```python
from build123d import *

# Parameters (mm, degrees)
BOSS_EXTRUDE1_DEPTH              = 6
FILLET1_R                        = 20
FILLET2_R                        = 20
SKETCH30_R                       = 10
CUT_EXTRUDE44_DEPTH              = 7
CUT_EXTRUDE44_DEPTH_BACK         = 1
SKETCH31_R                       = 5
CUT_EXTRUDE45_DEPTH              = 10
BODY_MOVE_COPY3_ANGLE            = 90
BODY_MOVE_COPY4_ANGLE            = 180
F_10_0MM_DOWEL_HOLE1_D           = 10
F_10_0MM_DOWEL_HOLE1_DEPTH       = 50
F_10_0MM_DOWEL_HOLE1_CSINK_D     = 10.05
F_10_0MM_DOWEL_HOLE1_CSINK_ANGLE = 90
F_10_0MM_DOWEL_HOLE1_TIP         = 3.004303095
SKETCH35_W                       = 43.4
SKETCH35_H                       = 43.4
CUT_EXTRUDE46_DEPTH              = 200


with BuildPart() as part:
    # Sketch6 → Boss-Extrude1 (new body)
    with BuildSketch(Plane.XY):
        Polygon((-61.363636364, 0), (61.363636364, 0), (90.231149823, -50), (90.231149823, -115), (54.237430104, -170), (54.237430104, -290), (-56.622130409, -290), (-56.622130409, -170), (-89.768850177, -115), (-89.768850177, -50), align=None)
    extrude(amount=BOSS_EXTRUDE1_DEPTH)

    # Fillet1
    fillet1_edges = [part.edges().sort_by_distance(p)[0] for p in [
        (54.237430104, -290, 3),
    ]]
    fillet(fillet1_edges, radius=FILLET1_R)

    # Fillet2
    fillet2_edges = [part.edges().sort_by_distance(p)[0] for p in [
        (-56.622130409, -290, 3),
    ]]
    fillet(fillet2_edges, radius=FILLET2_R)

    # Sketch30 → Cut-Extrude44 (cut, two sides)
    with BuildSketch(Plane.XY) as cut_extrude44_sk:
        with Locations((-1.192350152, -220)):
            Circle(SKETCH30_R)
    extrude(amount=CUT_EXTRUDE44_DEPTH, mode=Mode.SUBTRACT)
    extrude(cut_extrude44_sk.sketch, amount=-CUT_EXTRUDE44_DEPTH_BACK, mode=Mode.SUBTRACT)

    # Sketch31 → Cut-Extrude45 (cut)
    with BuildSketch(Plane.XY.offset(6)):
        with Locations((0, -69.133646514)):
            Circle(SKETCH31_R)
    extrude(amount=-CUT_EXTRUDE45_DEPTH, mode=Mode.SUBTRACT)


with BuildPart() as part_1:
    # Body-Move/Copy3: moved
    add(part.part.rotate(Axis((0, -121.936798964, -1), (1, 0, 0)), BODY_MOVE_COPY3_ANGLE))


with BuildPart() as part_2:
    # Body-Move/Copy4: moved
    add(part_1.part.rotate(Axis((0, -111.936798964, -21), (1, 0, 0)), BODY_MOVE_COPY4_ANGLE))


with BuildPart() as part_3:
    # Body-Move/Copy5: moved
    add(part_2.part.moved(Location((52.144140366, 0, 0))))

    # Ø10.0mm Dowel Hole1
    with Locations(Plane(origin=(0, -94.936798964, 0), x_dir=(1, 0, 0), z_dir=(0, 1, 0))):
        with Locations((51.761395867, -93.178073243)):
            CounterSinkHole(F_10_0MM_DOWEL_HOLE1_D / 2, F_10_0MM_DOWEL_HOLE1_CSINK_D / 2, depth=F_10_0MM_DOWEL_HOLE1_DEPTH, counter_sink_angle=F_10_0MM_DOWEL_HOLE1_CSINK_ANGLE)
            with Locations((0, 0, -(F_10_0MM_DOWEL_HOLE1_DEPTH + F_10_0MM_DOWEL_HOLE1_TIP / 2))):  # 118° drill point
                Cone(0, F_10_0MM_DOWEL_HOLE1_D / 2, F_10_0MM_DOWEL_HOLE1_TIP, mode=Mode.SUBTRACT)

    # Sketch35 → Cut-Extrude46 (cut)
    with BuildSketch(Plane(origin=(0, 0, 0), x_dir=(1, 0, 0), z_dir=(0, 1, 0))):
        with Locations((-5.062927598, 86.826541805)):
            Rectangle(SKETCH35_W, SKETCH35_H)
    extrude(amount=-CUT_EXTRUDE46_DEPTH, mode=Mode.SUBTRACT)


solid = part_3.part
```
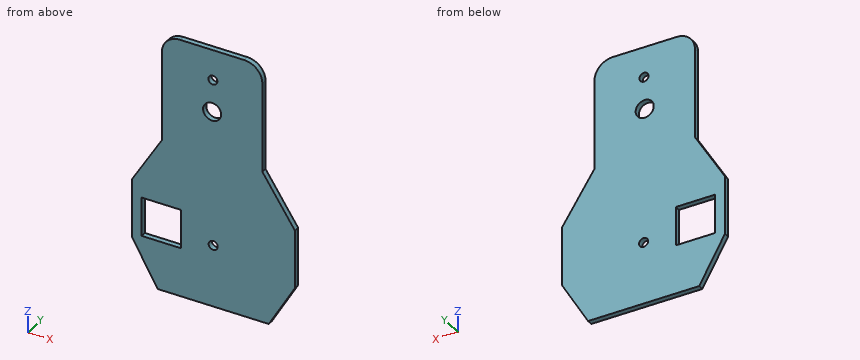
Here's how the part is built. I have some questions about the finished solid (model axes, mm). Coordinates: 2 decimals unless noted, no trailing zeros. Loops run counter-clockwise (first coordinate to the right, second up) from the corner with the lowest first, then second, coordinate; pieces in that order, holes last. Notation, with made-up numbers: (35.25, -35.75) -> (83.25, -35.75) arc R31 cw to (83.25, -0.75) -> close; hole circle Ø7 at (67.5, 74.5). An arc over 180 degrees is marked (long way). Return JSON: item names as keys, results as strings.
1) If we section it at A-A, the plane x = -1: Write out the boundary of the cut face in (y, z), then the cut area to 3 significant figures.
Results below:
{"outline": "(-100.94, -162.94) -> (-94.94, -162.94) -> (-94.94, -108.53) -> (-100.94, -108.53) -> close; (-100.94, -65.13) -> (-94.94, -65.13) -> (-94.94, 118.33) -> (-100.94, 118.33) -> close", "area": "1,430 mm²"}
2) If we section it at B-B, the plane y = -96.25: Write out the boundary of the cut face in (x, z).
Results below:
{"outline": "(-37.62, -112.94) -> (-9.22, -162.94) -> (113.51, -162.94) -> (142.38, -112.94) -> (142.38, -47.94) -> (106.38, 7.06) -> (106.38, 107.06) arc R20 ccw to (86.38, 127.06) -> (15.52, 127.06) arc R20 ccw to (-4.48, 107.06) -> (-4.48, 7.06) -> (-37.62, -47.94) -> close; hole (-26.76, -108.53) -> (16.64, -108.53) -> (16.64, -65.13) -> (-26.76, -65.13) -> close; hole circle Ø20 at (50.95, 57.06); hole circle Ø10 at (51.76, 93.18); hole circle Ø10 at (52.14, -93.8)"}
3) I need wall thicknesses on line 1 (X direction, y = -95, z = -93); line 2 (X direction, y = -95.25, z = 93); line 3 (X direction, y = -95.5, z = 24.5). Which ranges of each line are inside material? Lowest first, please. Write a range as from..to.
Results below:
{"line 1": "-37.62..-26.76, 16.64..47.21, 57.08..142.38", "line 2": "-4.48..46.76, 56.76..106.38", "line 3": "-4.48..106.38"}
4) If we section it at D-D, the plane z = -11: Write out the boundary of the cut face in (x, y), then the cut area to 3 significant figures.
Results below:
{"outline": "(-15.36, -100.94) -> (118.2, -100.94) -> (118.2, -94.94) -> (-15.36, -94.94) -> close", "area": "801 mm²"}
5) If we section it at C-C, the plane z = 42: Write out the boundary of the cut face in (x, y).
Results below:
{"outline": "(-4.48, -100.94) -> (106.38, -100.94) -> (106.38, -94.94) -> (-4.48, -94.94) -> close"}
6) Will these pins go through, and if not, where does the flat tip stop? pin 1 (1 mm diameter, centred on x = 89, y = -97, fed in from +Z); pin 2 (1.8 mm diameter, centred on y = -98.5, z = 42.5, fed in from +X); pin 3 (6 mm diameter, centred on x = 51.76, z = 93.18, fed in from -Y).
Results below:
{"pin 1": "z = 126.95", "pin 2": "x = 106.38", "pin 3": "through"}
